Geometry check sheet. Reference: the model listing, model coordinates, mm. A direction names the side the tool comes from. Round coordinates to 2 decimals unless told otherwise and drop trailing zeros. Write each loop counter-clockwise with the first axis right and the second up, starting at its lowest first coordinate (ties: lowest second). Pieces come first, ordered by that corner, then holes. Notation, with made-up numbers: M -19.5,80 L -14.5,80 A23 cw -14.5,118 Z; hole C -39.5,-16 d1. An arc over 180 degrees is marked long. Put each result on its own line as item: value. Start each with the question number.
(1) Material ranges on probe 1 along Y at (x, z) = (0, 57.85); probe 2 along Y at (x, z) = (0, 23); probe 3 along Z at (x, y) = (-16, 2.5), recorded low to high.
(2) Section check A-A on z = 26.5. Record the cut outline in (x, y), then the cut area to 3 significant figures.
(3) Section check D-D on y = -16.5. Record the cut outline in (x, z).
(4) Tool access check on faces 1 (the flat face through (18.6, 18.6, 1.2)), 2 (the flat face through (-8.3, 12.3, 0)). Record the directions out of +Z, -Z, +X, -X, +Y, -Y that give a thin tool (end or side, any length) a straight path to the whole face; none if there is none.
(5) Mould release check, pull along Y, two halves, no side actions. Record for faces 3 (the flat face through (19, -19, 30)), 4 (the cylindrical face through (-14.985, 0.66, 57.535)), 5 (the flat face through (0, 19, 1)): pulls with the +Y half, pulls with the -Y half, needs draft (parallel to the pull), parting line crosses it, or undercut.
(6) Section check B-B on x = 0. Record the cut outline in (y, z).
(7) Gauge pin test, flat end, axial feed: pin 1 (12 mm diameter, centred on x = 0, y = 0, fed in from +Z). Record the tip position at first contact, or that the pin passes through.
from build123d import *

# Parameters (mm, degrees)
F0_W     = 40
F0_H     = 40
F1_DEPTH = 60
F2_R     = 15
F3_DEPTH = 60
F5_START = -5
F4_R     = 15
F4_R_2   = 10
F5_DEPTH = 60
F6_SIZE  = 2
F7_W     = 88.496286422
F7_H     = 74.0717835724
F7_R     = 14.5
F8_DEPTH = 5


with BuildPart() as f1:
    # F0 (on Top) → F1 (new body)
    with BuildSketch(Plane.XY):
        Rectangle(F0_W, F0_H)
    extrude(amount=F1_DEPTH)

    # F2 (on face) → F3 (cut)
    with BuildSketch(Plane.XY.offset(60)):
        Circle(F2_R)
    extrude(amount=-F3_DEPTH, mode=Mode.SUBTRACT)

    # F4 (on face) → F5 (join)
    with BuildSketch(Plane.XY.offset(60).offset(F5_START)):
        Circle(F4_R)
        Circle(F4_R_2, mode=Mode.SUBTRACT)
    extrude(amount=-F5_DEPTH)

    # F6
    f6_edges = [f1.edges().sort_by_distance(p)[0] for p in [
        (20, -20, 30),
        (20, 20, 30),
        (-20, -20, 30),
        (20, 0, 60),
        (0, -20, 60),
        (-20, 0, 60),
        (0, 20, 60),
        (-20, 20, 30),
        (20, 0, 0),
        (0, -20, 0),
        (-20, 0, 0),
        (0, 20, 0),
    ]]
    chamfer(f6_edges, length=F6_SIZE)

    # F7 (on face) → F8 (cut)
    with BuildSketch(Plane(origin=(0, 0, -5), x_dir=(1, 0, 0), z_dir=(0, 0, -1))):
        with Locations((-0.5847793072, -3.7035886198)):
            Rectangle(F7_W, F7_H)
        Circle(F7_R, mode=Mode.SUBTRACT)
    extrude(amount=-F8_DEPTH, mode=Mode.SUBTRACT)


solid = f1.part
Answers follow:
1. probe 1: y = -20 to -15, 15 to 20
1. probe 2: y = -20 to -10, 10 to 20
1. probe 3: z = 0 to 60
2. outline: M -20,-18 L -18,-20 L 18,-20 L 20,-18 L 20,18 L 18,20 L -18,20 L -20,18 Z; hole C 0,0 d20
2. area: 1,280 mm^2
3. outline: M -20,2 L -18,0 L 18,0 L 20,2 L 20,58 L 18,60 L -18,60 L -20,58 Z
4. face 1: -Z, +X, +Y
4. face 2: -Z
5. face 3: pulls with the -Y half
5. face 4: undercut
5. face 5: pulls with the +Y half
6. outline: M -20,2 L -18,0 L -14.5,0 L -14.5,-5 L -10,-5 L -10,55 L -15,55 L -15,60 L -18,60 L -20,58 Z; M 10,-5 L 14.5,-5 L 14.5,0 L 18,0 L 20,2 L 20,58 L 18,60 L 15,60 L 15,55 L 10,55 Z
7. pin 1: passes through
